Read the model definition and answer for the solid it produces. Units are mm, in the model's axes. Face numbers are marked on the shaded views. A direction names the side the tool comes from. Give positions to 0.01 mm unless a question says otherwise; leave off trailing zeros. Order: outer loops, then holes, each group sorted by start corner. A loop starts at its lowest first (then second) coordinate and runs counter-clockwise, first axis right, second up. Notation, with made-up numbers: (62, 22) -> (75, 22) arc R19 cw to (75, 50) -> close; hole circle Ø1 at (31.5, 66.25). An arc over 180 degrees is marked (long way). Use one line per item in the form item = value.
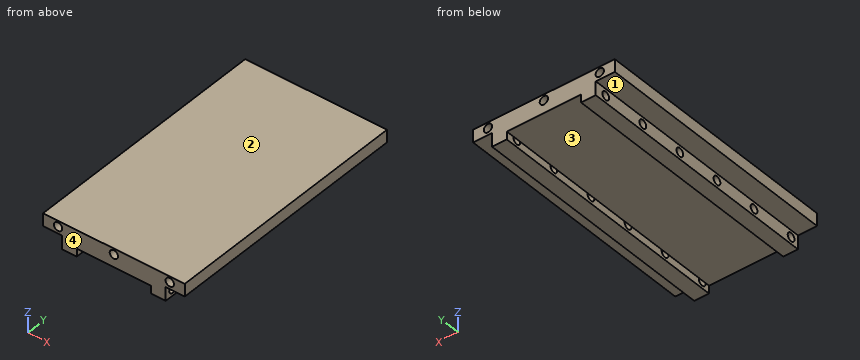
```python
from build123d import *

# Parameters (mm, degrees)
BOSS_EXTRUDE1_DEPTH = 300
SKETCH6_R           = 5
CUT_EXTRUDE2_DEPTH  = 17.67
SKETCH8_R           = 5
CUT_EXTRUDE3_DEPTH  = 10
CUT_EXTRUDE4_START  = -10
SKETCH9_R           = 5
CUT_EXTRUDE4_DEPTH  = 10


with BuildPart() as part:
    # Sketch2 → Boss-Extrude1 (new body)
    with BuildSketch(Plane(origin=(0, 0, 0), x_dir=(1, 0, 0), z_dir=(0, 1, 0))):
        Polygon((0, 0), (170, 0), (170, 15), (147.17, 15), (147.17, 31.396582403), (129.5, 31.396582403), (129.5, 22.061582403), (40.5, 22.061582403), (40.5, 31.396582403), (22.83, 31.396582403), (22.83, 15), (0, 15), align=None)
    extrude(amount=BOSS_EXTRUDE1_DEPTH)

    # Sketch6 → Cut-Extrude2 (cut)
    with BuildSketch(Plane(origin=(147.17, 0, 0), x_dir=(0, 0, -1), z_dir=(1, 0, 0))):
        with Locations((23.1975, 285.170960777)):
            Circle(SKETCH6_R)
        with Locations((23.1975, 230.170960777)):
            Circle(SKETCH6_R)
        with Locations((23.1975, 175.170960777)):
            Circle(SKETCH6_R)
        with Locations((23.1975, 120.170960777)):
            Circle(SKETCH6_R)
        with Locations((23.1975, 65.170960777)):
            Circle(SKETCH6_R)
        with Locations((23.1975, 10.170960777)):
            Circle(SKETCH6_R)
    cut_extrude2 = extrude(amount=-CUT_EXTRUDE2_DEPTH, mode=Mode.SUBTRACT)

    # Mirror1: Cut-Extrude2 across plane
    add(cut_extrude2.mirror(Plane.ZY.offset(-85)), mode=Mode.SUBTRACT)

    # Sketch8 → Cut-Extrude3 (cut)
    with BuildSketch(Plane(origin=(0, 300, 0), x_dir=(1, 0, 0), z_dir=(0, 1, 0))):
        with Locations(Location((152, 7.003164806, 0), (0, 0, 270))):
            Circle(SKETCH8_R)
        with Locations(Location((85, 7.003164806, 0), (0, 0, 270))):
            Circle(SKETCH8_R)
        with Locations(Location((18, 7.003164806, 0), (0, 0, 270))):
            Circle(SKETCH8_R)
    extrude(amount=-CUT_EXTRUDE3_DEPTH, mode=Mode.SUBTRACT)

    # Sketch9 → Cut-Extrude4 (cut)
    with BuildSketch(Plane.XZ.offset(CUT_EXTRUDE4_START)):
        with Locations(Location((18, -7.003164806, 0), (0, 0, 90))):
            Circle(SKETCH9_R)
        with Locations(Location((85, -7.003164806, 0), (0, 0, 90))):
            Circle(SKETCH9_R)
        with Locations(Location((152, -7.003164806, 0), (0, 0, 90))):
            Circle(SKETCH9_R)
    extrude(amount=CUT_EXTRUDE4_DEPTH, mode=Mode.SUBTRACT)


solid = part.part
```
Item 1: Determine the mould class of the marked faces 3 and 4 for opening direction X: +X half, -X half, draft (parallel to the pull), parting line (faces both ways), or undercut.
Checks:
face_3 = undercut
face_4 = draft
Item 2: The part is cut by section B-B on y = 81.5. Give the vertices of the cut face in (x, z), and give its area (3 significant figures).
Checks:
outline = (0, -15) -> (22.83, -15) -> (22.83, -31.4) -> (40.5, -31.4) -> (40.5, -22.06) -> (129.5, -22.06) -> (129.5, -31.4) -> (147.17, -31.4) -> (147.17, -15) -> (170, -15) -> (170, 0) -> (0, 0) -> close
area = 3,760 mm²
Item 3: Given pin 1 Ø4.5 at (y, z) = (77.5, -28.5) entering from +X; pin 2 Ø8 at (y, z) = (115.5, -27.5) entering from -X; pin 3 Ø11 at (x, z) = (18, -6) entering from -Y; pin 4 Ø1.2 at (y, z) = (174.5, -19.5) entering from -X, each flat-ended and moving along its own axis, determine where each tip first touches the part or whether it passes through.
Checks:
pin_1 = 147.17
pin_2 = 22.83
pin_3 = 0
pin_4 = 40.5
Item 4: The part is cut by section C-C on x = 53. Give the vertices of the cut face in (y, z), and give its area (3 significant figures).
Checks:
outline = (0, -22.06) -> (300, -22.06) -> (300, 0) -> (0, 0) -> close
area = 6,620 mm²
Item 5: Which of the six approach directions +Z, -Z, +X, -X, +Y, -Y give full straight-line access (tool end or side, diameter ignored) to the marked faces 1 and 2?
Checks:
face_1 = -Z, -X, +Y, -Y
face_2 = +Z, +X, -X, +Y, -Y
Item 6: The part is cut by section A-A on x = 152. Give the vertices of the cut face in (y, z).
Checks:
outline = (0, -15) -> (300, -15) -> (300, -12) -> (290, -12) -> (290, -2) -> (300, -2) -> (300, 0) -> (0, 0) -> (0, -2) -> (10, -2) -> (10, -12) -> (0, -12) -> close
Item 7: Straight lines are drawn through the part: L1, parallel to X at y = 45, z = -26.5; L2, parallel to Z at x = 116.5, y = 279; L3, parallel to Z at x = 154, y = 263.5. For each, find the intervals that lie inside material, in ascending order. Write a range as from..to.
Checks:
L1 = 22.83..40.5, 129.5..147.17
L2 = -22.06..0
L3 = -15..0
